Read the model definition and answer for the solid it produces. Units are mm, in the model's axes. Coordinates: 2 decimals unless noted, no trailing zeros. Loops run counter-clockwise (first coordinate to the right, second up) from the corner with the lowest first, then second, coordinate; pieces in that order, holes last. Notation, with made-up numbers: (55.5, 18.5) -> (96.5, 18.5) arc R12 cw to (96.5, 34.5) -> close; hole circle Ø6 at (-22.75, 59.25). An arc over 180 degrees is marked (long way). Answer as a JSON object with one key per item and string values. Group by question number.
Q1. The part is cut by section A-A on y = -3. Write down the section's boundary in (x, z) (3 decimals), and give its area (3 significant figures).
Q2. Straight lines are drawn through the part: line 1 along X through (y, z) = (-3.75, 20.5); line 2 along X through (y, z) = (-4.25, -9); line 3 along X through (y, z) = (-4.25, 24). For each, find the intervals that lie inside material, in ascending order. Write a range as [from, to].
Q3. Determine the mould class of faces 1 (the cylindrical face through (-60.8, -3.1, -23.3)), 2 (the flat face through (-1, -6.35, 1)), 3 (the cylindrical face through (57.618, -5.724, 8.106)) for opening direction X: released by +X, released by -X, zero draft, split by the parting line, or undercut.
Q4. The part is cut by section B-B on z = -11. State how many separate pieces and enclosed holes the cut face has, and give its area (3 significant figures).
Q5. Each of these flat-tipped pins is pushed along its axis until it touches: P1, Ø5, axis at x = 58.42, z = 25.4, coming from the +Y side; P2, Ø2, axis at x = 54.5, y = -5, coming from the -Z side; P3, Ø2, axis at y = -3.5, z = 9.5, coming from the +X side. Where does it stop, or does it pass through?
from build123d import *

# Parameters (mm, degrees)
F0_R     = 3.175
F1_DEPTH = 6.35
F2_DEPTH = 6.35
F4_R     = 26.9875
F5_DEPTH = 25.4


# Not quite as in the source:
# - a fillet or chamfer that OpenCascade refuses, or shapes differently, is made with other operations: its cross-section is extruded or revolved along the edge and cut away or added


with BuildPart() as f1:
    # F0 (on Front) → F1 (new body)
    with BuildSketch(Plane.XZ):
        with BuildLine():
            ThreePointArc((-76.2542010712, 0), (-65.0949694344, -26.9407683632), (-38.1542010712, -38.1))
            Line((-38.1542010712, -38.1), (38.0457989288, -38.1))
            ThreePointArc((38.0457989288, -38.1), (64.986567292, -26.9407683632), (76.1457989288, 0))
            ThreePointArc((76.1457989288, 0), (64.986567292, 26.9407683632), (38.0457989288, 38.1))
            Line((38.0457989288, 38.1), (-38.1542010712, 38.1))
            ThreePointArc((-38.1542010712, 38.1), (-65.0949694344, 26.9407683632), (-76.2542010712, 0))
        make_face()
        with Locations((-58.42, -25.4)):
            Circle(F0_R, mode=Mode.SUBTRACT)
        with Locations((58.42, -25.4)):
            Circle(F0_R, mode=Mode.SUBTRACT)
        with Locations((-58.42, 25.4)):
            Circle(F0_R, mode=Mode.SUBTRACT)
        with BuildLine():
            ThreePointArc((-31.75, -31.75), (-63.5, 0), (-31.75, 31.75))
            Line((-31.75, 31.75), (31.75, 31.75))
            ThreePointArc((31.75, 31.75), (63.5, 0), (31.75, -31.75))
            Line((31.75, -31.75), (-31.75, -31.75))
        make_face(mode=Mode.SUBTRACT)
        with Locations((58.42, 25.4)):
            Circle(F0_R, mode=Mode.SUBTRACT)
    extrude(amount=F1_DEPTH)

    # F0 (on Front) → F2 (join)
    with BuildSketch(Plane.XZ):
        with BuildLine():
            Line((31.75, 31.75), (-31.75, 31.75))
            ThreePointArc((-31.75, 31.75), (-63.5, 0), (-31.75, -31.75))
            Line((-31.75, -31.75), (31.75, -31.75))
            ThreePointArc((31.75, -31.75), (63.5, 0), (31.75, 31.75))
        make_face()
    extrude(amount=F2_DEPTH)

    # F4 (on face) → F5 (cut)
    with BuildSketch(Plane.XZ.offset(6.35)):
        with Locations((-31.877, 0)):
            Circle(F4_R)
        with Locations((31.877, 0)):
            Circle(F4_R)
    extrude(amount=-F5_DEPTH, mode=Mode.SUBTRACT)

    # F6: fillet of radius 5.08 on 2 edges, made by hand

    # F6_s1 → F6_t2 (revolve, cut)
    with BuildSketch(Plane.XY):
        with BuildLine():
            ThreePointArc((63.9445, 0), (60.3523975516, -1.4878975516), (58.8645, -5.08))
            Line((58.8645, -5.08), (58.8645, 0))
            Line((58.8645, 0), (63.9445, 0))
        make_face()
    revolve(axis=Axis((31.877, 0, 0), (0, -1, 0)), mode=Mode.SUBTRACT)

    # F6_s3 → F6_t4 (revolve, cut)
    with BuildSketch(Plane.XY):
        with BuildLine():
            ThreePointArc((0.1905, 0), (-3.4016024484, -1.4878975516), (-4.8895, -5.08))
            Line((-4.8895, -5.08), (-4.8895, 0))
            Line((-4.8895, 0), (0.1905, 0))
        make_face()
    revolve(axis=Axis((-31.877, 0, 0), (0, -1, 0)), mode=Mode.SUBTRACT)


solid = f1.part
Final values:
{
 "1": {"outline": "(-38.154, -38.1) -> (38.046, -38.1) arc R38.1 ccw to (38.046, 38.1) -> (-38.154, 38.1) arc R38.1 ccw to start; hole circle Ø6.35 at (-58.42, -25.4); hole circle Ø6.35 at (-58.42, 25.4); hole circle Ø54.866 at (-31.877, 0); hole circle Ø54.866 at (31.877, 0); hole circle Ø6.35 at (58.42, -25.4); hole circle Ø6.35 at (58.42, 25.4)", "area": "5,510 mm2"},
 "2": {"line 1": "x = [-70.27, -49.7], [-14.05, 14.05], [49.7, 70.16]", "line 2": "x = [-75.18, -57.39], [-6.36, 6.36], [57.39, 75.07]", "line 3": "x = [-67.74, -61.27], [-55.57, -44.37], [-19.39, 19.39], [44.37, 55.57], [61.27, 67.64]"},
 "3": {"face 1": "undercut", "face 2": "zero draft", "face 3": "undercut"},
 "4": {"separate pieces": "3", "enclosed holes": "0", "area": "297 mm2"},
 "5": {"P1": "passes through", "P2": "stops at z = -34.82", "P3": "stops at x = 75.19"}
}
